Could you check a few things on this model? Use its own coordinates, in mm. Give positions to 0.01 mm unless a question says otherwise; leave off trailing zeros. Loops run counter-clockwise (first coordinate to the right, second up) from the corner with the lowest first, then second, coordinate; pieces in that order, holes last. Notation, with made-up numbers: M 11.25,26 L 23.25,26 A23 ccw 23.25,58 Z; hole C 18.25,-21 d5. An arc over 180 degrees is marked long. Answer in a Markdown table with one row per item. Add a question column.
1. Thinking about a two-plate mould opening in X: for faces 1 (the cylindrical face through (-6.82, -7.56, 1.03)), 2 (the flat face through (0, 0, 0)), 3 (the cylindrical face through (-9.895, -7.587, 1.002)), which applies, released by +X, released by -X, zero draft, split by the parting line, or undercut?
2. If we section it at C-C on x = -3: List the corners of the cut face in (y, z) for me.
3. If we section it at B-B on z = 1.35: List the corners of the cut face in (x, y) for me.
4. I'm going to push a flat-ended pin straight in: pin 1 Ø2 at (x, y) = (6.09, 7.19) entering from -Z. Where does the tip first touch, or does it pass through?
5. If we section it at A-A on y = 7.75: List the corners of the cut face in (x, z) for me.
6. If we section it at D-D on y = 4.25: List the corners of the cut face in (x, z) for me, then the cut area to 3 significant figures.
7. I need wall thicknesses on line 1 along X through (y, z) = (6.5, 0.85); line 2 along Y through (x, z) = (-5, 0.6); line 3 along X through (y, z) = (7.25, 0.75). Which ranges of each line are inside material? Lowest first, please. Write a range as from..to.
```python
from build123d import *

# Parameters (mm, degrees)
F0_R     = 12.469473319
F2_DEPTH = 2.032
F3_D     = 2.54


with BuildPart() as f2:
    # F0 (on Top) → F2 (new body)
    with BuildSketch(Plane.XY):
        Circle(F0_R)
    extrude(amount=F2_DEPTH)

    # F3 (through all)
    with Locations(Plane(origin=(0, 0, 0), x_dir=(1, 0, 0), z_dir=(0, 0, -1))):
        with Locations((-5.6063276716, 7.1808281355), (6.5757827833, 7.4244700372), (6.0884971172, -7.1940617636), (-5.8499677107, -7.1940617636)):
            Hole(F3_D / 2)


solid = f2.part
```
Results:
| question | item | result |
|---|---|---|
| 1 | face 1 | undercut |
| 1 | face 2 | zero draft |
| 1 | face 3 | split by the parting line |
| 2 | outline | M -12.1,0 L 12.1,0 L 12.1,2.03 L -12.1,2.03 Z |
| 3 | outline | C 0,0 d24.94; hole C -5.85,7.19 d2.54; hole C -5.61,-7.18 d2.54; hole C 6.09,7.19 d2.54; hole C 6.58,-7.42 d2.54 |
| 4 | pin 1 | through |
| 5 | outline | M -9.77,0 L -6.99,0 L -6.99,2.03 L -9.77,2.03 Z; M -4.71,0 L 4.95,0 L 4.95,2.03 L -4.71,2.03 Z; M 7.23,0 L 9.77,0 L 9.77,2.03 L 7.23,2.03 Z |
| 6 | outline | M -11.72,0 L 11.72,0 L 11.72,2.03 L -11.72,2.03 Z |
| 6 | area | 47.6 mm2 |
| 7 | line 1 | -10.64..-6.91, -4.79..5.02, 7.15..10.64 |
| 7 | line 2 | -11.42..-8.3, -6.06..6.25, 8.14..11.42 |
| 7 | line 3 | -10.15..-7.12, -4.58..4.82, 7.36..10.15 |
